The listing builds one solid part. Answer for the finished solid, in the listing's coordinates (mm). Face numbers are marked on the shaded views. Give positions to 0.01 mm unless a question says otherwise; leave off trailing zeros. Order: outer loops, then holes, each group sorted by start corner. A loop starts at its lowest first (then second) coordinate and runs counter-clockwise, first axis right, second up.
```python
from build123d import *

# Parameters (mm, degrees)
CYLINDER024_R     = 8
CYLINDER024_DEPTH = 10
ARRAY003_COUNT    = 5
CYLINDER023_R     = 1.5
CYLINDER023_DEPTH = 10
TORUS005_R        = 0.8
TORUS004_R        = 0.8
CYLINDER021_R     = 30
CYLINDER021_DEPTH = 5
CYLINDER022_R     = 3
CYLINDER022_DEPTH = 10


with BuildPart() as fusion014:
    # Cylinder024 → Cylinder024 (new body)
    with BuildSketch(Plane(origin=(0, 15, 0), x_dir=(1, 0, 0), z_dir=(0, 0, 1))):
        Circle(CYLINDER024_R)
    extrude(amount=CYLINDER024_DEPTH)

    # Array003: Fusion014 ×5 about axis
    array003_axis = Axis((0, 0, 0), (0, 0, 1))


with BuildPart() as fusion014_1:
    add(fusion014.part)
    for i in range(1, ARRAY003_COUNT):
        add(fusion014.part.rotate(array003_axis, i * 360 / ARRAY003_COUNT))


with BuildPart() as cylinder023:
    # Cylinder023 → Cylinder023 (new body)
    with BuildSketch(Plane.XY):
        Circle(CYLINDER023_R)
    extrude(amount=CYLINDER023_DEPTH)


with BuildPart() as torus005:
    # Torus005 → Torus005 (revolve)
    with BuildSketch(Plane(origin=(0, 0, 3.5), x_dir=(1, 0, 0), z_dir=(0, -1, 0))):
        with Locations((30, 0)):
            Circle(TORUS005_R)
    revolve(axis=Axis((0, 0, 3.5), (0, 0, 1)))


with BuildPart() as torus004:
    # Torus004 → Torus004 (revolve)
    with BuildSketch(Plane(origin=(0, 0, 1.5), x_dir=(1, 0, 0), z_dir=(0, -1, 0))):
        with Locations((30, 0)):
            Circle(TORUS004_R)
    revolve(axis=Axis((0, 0, 1.5), (0, 0, 1)))


with BuildPart() as cut015:
    # Cylinder021 → Cylinder021 (new body)
    with BuildSketch(Plane.XY):
        Circle(CYLINDER021_R)
    extrude(amount=CYLINDER021_DEPTH)

    # Cut014: cut Torus004
    add(torus004.part, mode=Mode.SUBTRACT)

    # Cut015: cut Torus005
    add(torus005.part, mode=Mode.SUBTRACT)


with BuildPart() as cut017:
    # Cylinder022 → Cylinder022 (new body)
    with BuildSketch(Plane.XY):
        Circle(CYLINDER022_R)
    extrude(amount=CYLINDER022_DEPTH)

    # Fusion013: union Cut015
    add(cut015.part)

    # Cut016: cut Cylinder023
    add(cylinder023.part, mode=Mode.SUBTRACT)

    # Cut017: cut Fusion014
    add(fusion014_1.part, mode=Mode.SUBTRACT)


with BuildPart() as cut017_1:
    # Cut017 placement: moved
    add(cut017.part.moved(Location((47, 54, -26))))


solid = cut017_1.part
```
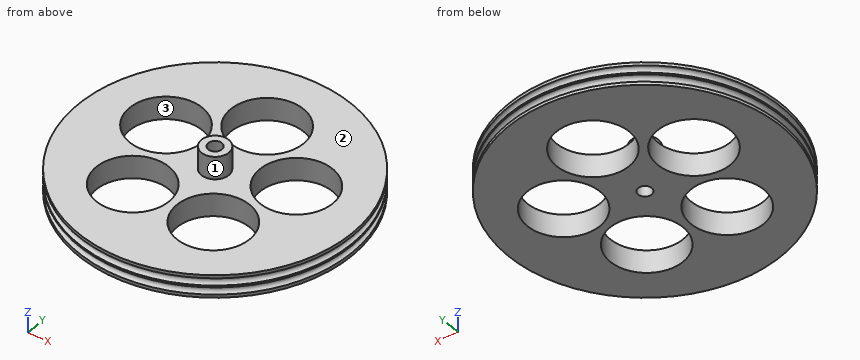
1) Find section A-A (x = 47). Write down the section's boundary in (y, z), then the cut area to 3 significant figures.
Geometry says:
outline: (24, -26) - (52.5, -26) - (52.5, -16) - (51, -16) - (51, -21) - (24, -21) - (24, -21.7) arc R0.8 cw to (24, -23.3) - (24, -23.7) arc R0.8 cw to (24, -25.3) - close; (55.5, -26) - (61, -26) - (61, -21) - (57, -21) - (57, -16) - (55.5, -16) - close; (77, -26) - (84, -26) - (84, -25.3) arc R0.8 cw to (84, -23.7) - (84, -23.3) arc R0.8 cw to (84, -21.7) - (84, -21) - (77, -21) - close
area: 216 mm2
2) Straight lines are drawn through the part: probe 1 along Z at (x, y) = (75.5, 46.5); probe 2 along Y at (x, z) = (63, -22.5); probe 3 along Y at (x, z) = (46, -16.25). For each, find the intervals that lie inside material, in ascending order.
Geometry says:
probe 1: z = -26 to -25.1, -23.9 to -23.1, -21.9 to -21
probe 2: y = 29.57 to 38.34, 45.39 to 50.83, 66.45 to 78.43
probe 3: y = 51.17 to 52.88, 55.12 to 56.83
3) Find section D-D (z = -18.5). Write down the section's boundary in (x, y).
Geometry says:
outline: circle Ø6 at (47, 54); hole circle Ø3 at (47, 54)
4) Given P1, Ø5, axis at x = 40, z = -20, coming from the +Y side; P2, Ø5, axis at x = 46.5, z = -24.5, coming from the +Y side; P3, Ø18.5, axis at x = 32.73, y = 58.64, coming from the +Z side, each flat-ended and moving along its own axis, determine where each tip first touches the part or whether it passes through.
Geometry says:
P1: stops at y = 83.63
P2: stops at y = 84
P3: stops at z = -21
5) Find section B-B (z = -22.5). Write down the section's boundary in (x, y), then the cut area to 3 significant figures.
Geometry says:
outline: circle Ø58.4 at (47, 54); hole circle Ø16 at (32.73, 58.64); hole circle Ø16 at (38.18, 41.86); hole circle Ø16 at (47, 69); hole circle Ø3 at (47, 54); hole circle Ø16 at (55.82, 41.86); hole circle Ø16 at (61.27, 58.64)
area: 1,670 mm2
6) For a pull along X with two mould halves and no side action, classify the marked faces 1, 2 and 3 as +X half, -X half, draft (parallel to the pull), parting line (faces both ways), or undercut.
Geometry says:
face 1: parting line
face 2: draft
face 3: undercut
7) Find section C-C (y = 54). Write down the section's boundary in (x, z), then the cut area to 3 significant figures.
Geometry says:
outline: (17, -26) - (26.21, -26) - (26.21, -21) - (17, -21) - (17, -21.7) arc R0.8 cw to (17, -23.3) - (17, -23.7) arc R0.8 cw to (17, -25.3) - close; (39.25, -26) - (45.5, -26) - (45.5, -16) - (44, -16) - (44, -21) - (39.25, -21) - close; (48.5, -26) - (54.75, -26) - (54.75, -21) - (50, -21) - (50, -16) - (48.5, -16) - close; (67.79, -26) - (77, -26) - (77, -25.3) arc R0.8 cw to (77, -23.7) - (77, -23.3) arc R0.8 cw to (77, -21.7) - (77, -21) - (67.79, -21) - close
area: 166 mm2
